Autodesk Inventor part; units mm, degrees
ref_plane "YZ Plane" through (0, 0, 0) normal (1, 0, 0) x (0, 1, 0)
ref_plane "XZ Plane" through (0, 0, 0) normal (0, 1, 0) x (-1, 0, 0)
ref_plane "XY Plane" through (0, 0, 0) normal (0, 0, 1) x (1, 0, 0)
sketch "Sketch1" plane through (0, 0, 0) normal (0, 0, 1) x (1, 0, 0)
  line L0 (-187.4297, 132.1193) -> (307.8703, 132.1193)
  line L1 (307.8703, 132.1193) -> (307.8703, 81.3193)
  line L2 (307.8703, 81.3193) -> (-187.4297, 81.3193)
  line L3 (-187.4297, 81.3193) -> (-187.4297, 132.1193)
  point P0 (0, 0)
  dimension "d0" = 495.3
  dimension "d1" = 50.8
extrude "Extrusion1" add sketch "Sketch1" along normal blind 25.4
sketch "Sketch2" plane through (-187.4297, 132.1193, 0) normal (0, 1, 0) x (1, 0, 0)
  circle A0 centre (12.7, -12.7) radius 2.5019
  line L0 (0, 0) -> (0, -25.4)
  circle A1 centre (25.4, -12.7) radius 2.5019
  circle A2 centre (38.1, -12.7) radius 2.5019
  circle A3 centre (482.6, -12.7) radius 2.5019
  line L1 (495.3, 0) -> (495.3, -25.4)
  circle A4 centre (469.9, -12.7) radius 2.5019
  circle A5 centre (457.2, -12.7) radius 2.5019
  circle A6 centre (368.3, -12.7) radius 2.5527
  circle A7 centre (247.65, -12.7) radius 3.9751
  line L2 (495.3, 0) -> (0, 0)
  circle A8 centre (127, -12.7) radius 2.5527
  point P0 (187.4297, 0)
  dimension "d4" = 12.7
  dimension "d5" = 5.0038
  dimension "d6" = 5.0038
  dimension "d7" = 5.0038
  dimension "d8" = 12.7
  dimension "d9" = 12.7
  dimension "d10" = 5.0038
  dimension "d11" = 12.7
  dimension "d12" = 5.0038
  dimension "d13" = 5.0038
  dimension "d14" = 12.7
  dimension "d15" = 12.7
  dimension "d19" = 127
  dimension "d20" = 5.1054
  dimension "d23" = 7.9502
  dimension "d24" = 247.65
  dimension "d25" = 12.7
  dimension "d26" = 5.1054
  dimension "d27" = 127
extrude "Extrusion2" cut sketch "Sketch2" against normal blind 50.8
shell "Shell1" thickness 3.175 removed faces 8 at (-187.4297, 115.186, 16.9333) at (307.8703, 98.2527, 8.4667) at (295.0696, 98.2527, 10.2001) at (282.3696, 98.2527, 10.2001) at (269.6696, 98.2527, 10.2001) at (-149.4304, 98.2527, 10.2001) at (-162.1304, 98.2527, 10.2001) at (-174.8304, 98.2527, 10.2001)
properties part number "(b)swerveassembly" material "Aluminum 6061"
Work out the finished part from the listing and answer in its coordinate system (mm). A direction names the side the tool comes from. Round coordinates to 2 decimals unless told otherwise and drop trailing zeros. Write each loop counter-clockwise with the first axis right and the second up, starting at its lowest first coordinate (ties: lowest second). Pieces come first, ordered by that corner, then holes. Notation, with made-up numbers: (89.25, 41.25) - (146.25, 41.25) arc R16 ccw to (146.25, 71.25) - close; hole circle Ø3 at (70, 19). An arc over 180 degrees is marked (long way). Answer in a Markdown table with one row per item. Add a question column.
1. The mould has two halves that part along Y. Classify faces 4 (the flat face through (56.8, 132.119, 15.3)), 5 (the flat face through (64, 84.494, 6)), 6 (the cylindrical face through (64.012, 107.075, 11.506)): +Y half, -Y half, draft (parallel to the pull), parting line (faces both ways), or undercut.
2. Given pin 1 (1.5 mm diameter, centred on y = 124.5, z = 13.5, fed in from +X); pin 2 (5 mm diameter, centred on y = 94.5, z = 7, fed in from -X), each flat-ended and moving along its own axis, determine where each tip first touches the part or whether it passes through.
3. A cutting plane is placed at A-A, the plane y = 92. Determine the outline of the cut face in (x, z) (3 decimals).
4. A cutting plane is placed at B-B, the plane x = 162. Determine the outline of the cut face in (y, z) (3 decimals), and give its area (3 significant figures).
5. For faces 1 (the flat face through (57, 107, 3.175)), 2 (the cylindrical face through (-55.139, 107.03, 14.894)), 3 (the flat face through (-187.43, 107, 2)), determine the directions among +Z, -Z, +X, -X, +Y, -Y from which every point of the face is accessible in a straight line to the end or side of a thin tool.
6. Find the intervals of material crossed by line 1 along X through (y, z) = (119, 12.7); line 2 along Y through (x, z) = (194.5, 4.25); line 3 along Z through (x, y) = (254.5, 118) (3 decimals), in increasing order. Write a range as from..to.
Worked out:
| question | item | result |
|---|---|---|
| 1 | face 4 | +Y half |
| 1 | face 5 | undercut |
| 1 | face 6 | draft |
| 2 | pin 1 | x = 186.6 |
| 2 | pin 2 | x = -65.18 |
| 3 | outline | (-187.43, 0) - (307.87, 0) - (307.87, 3.175) - (-187.43, 3.175) - close; (-187.43, 22.225) - (307.87, 22.225) - (307.87, 25.4) - (-187.43, 25.4) - close; circle Ø11.455 at (-60.43, 12.7); circle Ø14.3 at (60.22, 12.7); circle Ø11.455 at (180.87, 12.7); hole circle Ø5.105 at (-60.43, 12.7); hole circle Ø7.95 at (60.22, 12.7); hole circle Ø5.105 at (180.87, 12.7) |
| 4 | outline | (81.319, 0) - (132.119, 0) - (132.119, 25.4) - (81.319, 25.4) - close; hole (84.494, 3.175) - (128.944, 3.175) - (128.944, 22.225) - (84.494, 22.225) - close |
| 4 | area | 444 mm^2 |
| 5 | face 1 | +X, -X |
| 5 | face 2 | none |
| 5 | face 3 | +Z, -Z, -X, +Y, -Y |
| 6 | line 1 | -66.16..-62.98, -57.88..-54.7, 53.07..56.25, 64.2..67.37, 175.14..178.32, 183.42..186.6 |
| 6 | line 2 | 81.32..84.49, 128.94..132.12 |
| 6 | line 3 | 0..3.175, 22.225..25.4 |
